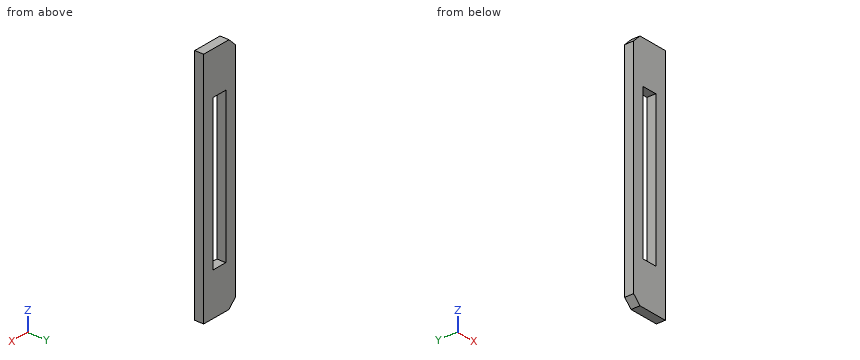
Autodesk Inventor part; units mm, degrees
ref_plane "YZ Plane" through (0, 0, 0) normal (1, 0, 0) x (0, 1, 0)
ref_plane "XZ Plane" through (0, 0, 0) normal (0, 1, 0) x (-1, 0, 0)
ref_plane "XY Plane" through (0, 0, 0) normal (0, 0, 1) x (1, 0, 0)
sketch "Sketch1" plane through (0, 0, 0) normal (0, 1, 0) x (-1, 0, 0)
  line L0 (-1.25, -7.9) -> (1.25, -7.9)
  line L1 (1.25, -7.9) -> (1.25, 7.9)
  line L2 (1.25, 7.9) -> (-1.25, 7.9)
  line L3 (-1.25, 7.9) -> (-1.25, -7.9)
  point P0 (0, 0)
  dimension "d0" = 15.8
  dimension "d7" = 1.25
  dimension "d8" = 1.25
extrude "Extrusion1" add sketch "Sketch1" along normal blind 0.6
sketch "Sketch2" plane through (0, 0.6, 0) normal (0, 1, 0) x (1, 0, 0)
  line L0 (0.5, 5.05) -> (-0.5, 5.05)
  line L1 (-0.5, 5.05) -> (-0.5, -5.05)
  line L2 (-0.5, -5.05) -> (0.5, -5.05)
  line L3 (0.5, -5.05) -> (0.5, 5.05)
  line L4 (0.5, 5.05) -> (-0.5, -5.05) construction
  line L5 (-0.5, 5.05) -> (0.5, -5.05) construction
  point P0 (0, 0)
  dimension "d3" = 1
  dimension "d4" = 10.1
extrude "Extrusion2" cut sketch "Sketch2" against normal through all
sketch "Sketch3" plane through (0, 0.6, 0) normal (0, 1, 0) x (1, 0, 0)
  line L0 (-1.25, 7.9) -> (-1.25, -7.9)
  line L1 (-1.25, -7.4) -> (-0.75, -7.9)
  line L2 (-1.25, -7.9) -> (1.25, -7.9)
  line L3 (1.25, 7.9) -> (-1.25, 7.9)
  line L4 (-1.25, 7.4) -> (-0.75, 7.9)
  point P0 (0, 0)
  dimension "d9" = 0.5
  dimension "d10" = 0.5
  dimension "d11" = 0.5
  dimension "d12" = 0.5
extrude "Extrusion3" cut sketch "Sketch3" against normal through all
properties part number "insert spacer - v3"
Here's how the part is built. I have some questions about the finished solid (model axes, mm). Give positions to 0.01 mm unless a question says otherwise; leave off trailing zeros. Order: outer loops, then holes, each group sorted by start corner. A loop starts at its lowest first (then second) coordinate and runs counter-clockwise, first axis right, second up. Notation, with made-up numbers: M 85,-8 L 117,-8 A37 ccw 117,31 Z; hole C 3,-35 d8. An arc over 180 degrees is marked long. Use a Markdown table: item, result. Add a question column.
1. Suppose I cut it at B-B (y = 0.25). List the corners of the cut face in (x, z) for me, and give its area (4 significant figures).
2. I need wall thicknesses on probe 1 along X at (y, z) = (0.5, -2.5); probe 2 along Z at (x, y) = (0.2, 0.1); probe 3 along Z at (x, y) = (-0.8, 0.1). Which ranges of each line are inside material? Lowest first, please. Write a range as from..to.
3. For pin 1 Ø1.5 at (x, z) = (0, -2) entering from -Y, with a flat end and sliding along its axis, tell me the tip position at first contact or that it passes through.
4. Suppose I cut it at C-C (x = 0.25). List the corners of the cut face in (y, z) for me.
5. Suppose I cut it at A-A (z = -1.25). List the corners of the cut face in (x, y) for me, and give its area (3 significant figures).
Results list:
| question | item | result |
|---|---|---|
| 1 | outline | M -1.25,-7.4 L -0.75,-7.9 L 1.25,-7.9 L 1.25,7.9 L -0.75,7.9 L -1.25,7.4 Z; hole M -0.5,-5.05 L 0.5,-5.05 L 0.5,5.05 L -0.5,5.05 Z |
| 1 | area | 29.15 mm² |
| 2 | probe 1 | x = -1.25..-0.5, 0.5..1.25 |
| 2 | probe 2 | z = -7.9..-5.05, 5.05..7.9 |
| 2 | probe 3 | z = -7.85..7.85 |
| 3 | pin 1 | stops at y = 0 |
| 4 | outline | M 0,-7.9 L 0.6,-7.9 L 0.6,-5.05 L 0,-5.05 Z; M 0,5.05 L 0.6,5.05 L 0.6,7.9 L 0,7.9 Z |
| 5 | outline | M -1.25,0 L -0.5,0 L -0.5,0.6 L -1.25,0.6 Z; M 0.5,0 L 1.25,0 L 1.25,0.6 L 0.5,0.6 Z |
| 5 | area | 0.900 mm² |
